Here's how the part is built. I have some questions about the finished solid (model axes, mm). Coordinates: 2 decimals unless noted, no trailing zeros. Write each loop counter-clockwise with the first axis right and the second up, starting at its lowest first coordinate (ties: lowest second). Pieces come first, ordered by that corner, then holes. Notation, with made-up numbers: (-39.5, 1) -> (-20.5, 1) arc R29 cw to (-20.5, 24) -> close; hole circle Ø8 at (-8, 22). An arc over 180 degrees is marked (long way). Answer in a Markdown table with one row per item. Add a question column.
from build123d import *

# Parameters (mm, degrees)
SKETCH2_R           = 125.73
BOSS_EXTRUDE1_DEPTH = 6.35
SKETCH3_R           = 5.7546875
SKETCH3_R_2         = 26.67
CUT_EXTRUDE1_DEPTH  = 6.35


with BuildPart() as part:
    # Sketch2 → Boss-Extrude1 (new body)
    with BuildSketch(Plane(origin=(0, 0, 0), x_dir=(1, 0, 0), z_dir=(0, 1, 0))):
        with Locations(Location((0, 0, 0), (0, 0, 270))):
            Circle(SKETCH2_R)
    extrude(amount=BOSS_EXTRUDE1_DEPTH)

    # Sketch3 → Cut-Extrude1 (cut)
    with BuildSketch(Plane(origin=(0, 6.35, 0), x_dir=(1, 0, 0), z_dir=(0, 1, 0))):
        with Locations(Location((4.9245e-05, 39.6875, 0), (0, 0, 270))):
            Circle(SKETCH3_R)
        with Locations(Location((39.687549245, 0, 0), (0, 0, 270))):
            Circle(SKETCH3_R)
        with Locations(Location((4.9245e-05, -39.6875, 0), (0, 0, 270))):
            Circle(SKETCH3_R)
        with Locations(Location((-39.687450755, 0, 0), (0, 0, 270))):
            Circle(SKETCH3_R)
        with Locations(Location((0, 0, 0), (0, 0, 270))):
            Circle(SKETCH3_R_2)
        with BuildLine():
            Line((-4.7625, 107.85348), (-4.7625, 116.74348))
            ThreePointArc((-4.7625, 116.74348), (0, 121.50598), (4.7625, 116.74348))
            Line((4.7625, 116.74348), (4.7625, 107.85348))
            ThreePointArc((4.7625, 107.85348), (0, 103.09098), (-4.7625, 107.85348))
        make_face()
        with BuildLine():
            Line((107.853529245, 4.762549245), (116.743529245, 4.762549245))
            ThreePointArc((116.743529245, 4.762549245), (121.506029245, 4.9245e-05), (116.743529245, -4.762450755))
            Line((116.743529245, -4.762450755), (107.853529245, -4.762450755))
            ThreePointArc((107.853529245, -4.762450755), (103.091029245, 4.9245e-05), (107.853529245, 4.762549245))
        make_face()
        with BuildLine():
            Line((4.762598491, -107.85348), (4.762598491, -116.74348))
            ThreePointArc((4.762598491, -116.74348), (9.8491e-05, -121.50598), (-4.762401509, -116.74348))
            Line((-4.762401509, -116.74348), (-4.762401509, -107.85348))
            ThreePointArc((-4.762401509, -107.85348), (9.8491e-05, -103.09098), (4.762598491, -107.85348))
        make_face()
        with BuildLine():
            Line((-107.853430755, -4.762549245), (-116.743430755, -4.762549245))
            ThreePointArc((-116.743430755, -4.762549245), (-121.505930755, -4.9245e-05), (-116.743430755, 4.762450755))
            Line((-116.743430755, 4.762450755), (-107.853430755, 4.762450755))
            ThreePointArc((-107.853430755, 4.762450755), (-103.090930755, -4.9245e-05), (-107.853430755, -4.762549245))
        make_face()
    extrude(amount=-CUT_EXTRUDE1_DEPTH, mode=Mode.SUBTRACT)


solid = part.part
Q1. If we mould it in two halves opening along X, with no side actions, what happens to faces 1 (the cylindrical face through (0.105, 3.219, 121.505)), 2 (the cylindrical face through (-76.5, 3.13, -99.78)), 3 (the cylindrical face through (121.505, 3.219, -0.105)), 4 (the flat face through (30, 6.35, -2))? For each: pulls with the +X half, pulls with the -X half, needs draft (parallel to the pull), parting line crosses it, or undercut.
Q2. Imagine slicing it at A-A on z = 0. Please give me the cut outline in (x, y), plus the area to 3 significant figures.
Q3. Imagine slicing it at B-B on y = 4.5. State how many separate pieces and enclosed holes the cut face has, plus the area to 3 significant figures.
Q4. I'm going to push flat-ended pins straight in: P1, Ø3, axis at x = 111.5, y = 4.5, coming from the -Z side; P2, Ø13, axis at x = 0, z = -39.69, coming from the +Y side; P3, Ø1.9, axis at x = -114, y = 4.5, coming from the +Z side; P4, Ø1.9, axis at y = 2, z = -111.5, coming from the -X side. Where does each tip first touch, or does it pass through?
Q5. I need wall thicknesses on line 1 (X direction, y = 4.5, z = 0); line 2 (Z direction, x = -2, y = 5.75); line 3 (Z direction, x = 17, y = 4.25). Which ranges of each line are inside material? Lowest first, please. Write a range as [from, to].
Q6. Imagine slicing it at D-D on z = 61.5. Please give me the cut outline in (x, y), plus the area to 3 significant figures.
Q7. Imagine slicing it at C-C on x = -100. Please give me the cut outline in (y, z).
Result sheet:
| question | item | result |
|---|---|---|
| 1 | face 1 | undercut |
| 1 | face 2 | parting line crosses it |
| 1 | face 3 | undercut |
| 1 | face 4 | needs draft |
| 2 | outline | (-125.73, 0) -> (-121.51, 0) -> (-121.51, 6.35) -> (-125.73, 6.35) -> close; (-103.09, 0) -> (-45.44, 0) -> (-45.44, 6.35) -> (-103.09, 6.35) -> close; (-33.93, 0) -> (-26.67, 0) -> (-26.67, 6.35) -> (-33.93, 6.35) -> close; (26.67, 0) -> (33.93, 0) -> (33.93, 6.35) -> (26.67, 6.35) -> close; (45.44, 0) -> (103.09, 0) -> (103.09, 6.35) -> (45.44, 6.35) -> close; (121.51, 0) -> (125.73, 0) -> (125.73, 6.35) -> (121.51, 6.35) -> close |
| 2 | area | 878 mm^2 |
| 3 | separate pieces | 1 |
| 3 | enclosed holes | 9 |
| 3 | area | 46,400 mm^2 |
| 4 | P1 | stops at z = -60.89 |
| 4 | P2 | stops at y = 6.35 |
| 4 | P3 | stops at z = 55.02 |
| 4 | P4 | stops at x = -59.89 |
| 5 | line 1 | x = [-125.73, -121.51], [-103.09, -45.44], [-33.93, -26.67], [26.67, 33.93], [45.44, 103.09], [121.51, 125.73] |
| 5 | line 2 | z = [-125.71, -121.07], [-103.53, -45.08], [-34.29, -26.59], [26.59, 34.29], [45.08, 103.53], [121.07, 125.71] |
| 5 | line 3 | z = [-124.58, -20.55], [20.55, 124.58] |
| 6 | outline | (-109.66, 0) -> (109.66, 0) -> (109.66, 6.35) -> (-109.66, 6.35) -> close |
| 6 | area | 1,390 mm^2 |
| 7 | outline | (0, -76.21) -> (6.35, -76.21) -> (6.35, 76.21) -> (0, 76.21) -> close |
